Source: CAD feature listing. Evaluate the final solid. Frame: model axes, mm. A direction names the side the tool comes from. Round coordinates to 2 decimals unless told otherwise and drop trailing zeros. Loops run counter-clockwise (first coordinate to the right, second up) from the corner with the lowest first, then second, coordinate; pieces in that order, holes last. Notation, with made-up numbers: (49.5, 84) -> (57.5, 84) arc R23 cw to (57.5, 103) -> close; hole circle Ø10 at (10, 83.25). An arc over 180 degrees is marked (long way). Write item = value, one per line.
Autodesk Inventor part; units mm, degrees
ref_plane "YZ Plane" through (0, 0, 0) normal (1, 0, 0) x (0, 1, 0)
ref_plane "XZ Plane" through (0, 0, 0) normal (0, 1, 0) x (-1, 0, 0)
ref_plane "XY Plane" through (0, 0, 0) normal (0, 0, 1) x (1, 0, 0)
sketch "Sketch1" plane through (0, 0, 0) normal (0, 0, 1) x (1, 0, 0)
  line L0 (-121.92, 53.34) -> (121.92, 53.34)
  line L1 (121.92, 53.34) -> (121.92, -53.34)
  line L2 (121.92, -53.34) -> (-121.92, -53.34)
  line L3 (-121.92, -53.34) -> (-121.92, 53.34)
  line L4 (-121.92, 53.34) -> (121.92, -53.34) construction
  line L5 (121.92, 53.34) -> (-121.92, -53.34) construction
  line L6 (99.0307, 67.3864) -> (98.1801, -71.8373) construction
  line L7 (98.1801, -71.8373) -> (-108.1272, -70.5768) construction
  line L8 (-108.1272, -70.5768) -> (-107.2765, 68.6469) construction
  line L9 (-107.2765, 68.6469) -> (99.0307, 67.3864) construction
  arc A0 (-78.8873, -40.6173) -> (-95.4767, -51.4852) centre (-84.9112, -49.5176) ccw
  arc A1 (-78.8873, -40.6173) -> (-56.3395, -33.0982) centre (-70.4947, -28.2175) ccw
  arc A2 (-36.1227, -22.9374) -> (-56.3395, -33.0982) centre (-42.6558, -35.1316) ccw
  arc A3 (-19.5186, -13.8085) -> (-36.1227, -22.9374) centre (-17.295, -37.5173) ccw
  arc A4 (-68.7224, -13.6289) -> (-40.5344, -17.4333) centre (-51.1537, 10.214) ccw
  arc A5 (-68.7224, -13.6289) -> (-83.4187, -26.4721) centre (-67.6747, -29.6577) ccw
  arc A6 (-92.1839, -37.2444) -> (-83.4187, -26.4721) centre (-103.1345, -19.3818) ccw
  arc A7 (-92.1839, -37.2444) -> (-99.3105, -45.0028) centre (-83.147, -52.6977) ccw
  arc A8 (-99.3105, -45.0028) -> (-95.4767, -51.4852) centre (-95.2121, -46.9539) ccw
  arc A9 (-82.2314, -34.4993) -> (-57.5296, -25.5657) centre (-70.7814, -27.5415) ccw
  arc A10 (-57.5296, -25.5657) -> (-82.2314, -34.4993) centre (-69.6152, -30.7661) ccw
  line L10 (5.4328, -6.7323) -> (-19.5186, -13.8085)
  line L11 (5.4328, -6.7323) -> (85.4483, -20.8459)
  line L12 (85.4483, -20.8459) -> (85.8807, -18.3941)
  line L13 (85.8807, -18.3941) -> (26.167, -0.0762)
  line L14 (26.167, -0.0762) -> (86.2931, 21.1025)
  line L15 (86.2931, 21.1025) -> (85.711, 23.1551)
  arc A11 (85.711, 23.1551) -> (3.7291, 6.4763) centre (298.902, -1234.5808) ccw
  line L16 (-54.4933, 26.4309) -> (-67.6017, 26.4309)
  line L17 (-67.6017, 26.4309) -> (-72.6264, 27.9793)
  line L18 (-72.6264, 27.9793) -> (-69.6152, 32.3411)
  line L19 (-69.6152, 32.3411) -> (-69.6152, 41.676)
  arc A12 (-43.7838, 43.5271) -> (-69.6152, 41.676) centre (-56.4305, 38.848) ccw
  arc A13 (-47.6138, 46.2719) -> (-67.6017, 37.0085) centre (-56.174, 38.5465) ccw
  arc A14 (-67.6017, 37.0085) -> (-47.6138, 46.2719) centre (-56.6407, 39.5536) ccw
  arc A15 (-42.5631, 37.0085) -> (-43.7838, 43.5271) centre (-53.7825, 38.2811) ccw
  arc A16 (-42.5631, 37.0085) -> (-34.9749, 24.888) centre (-24.5395, 39.8568) ccw
  line L20 (-54.4933, 26.4309) -> (-47.0393, 26.4309)
  arc A17 (-36.0743, 21.1026) -> (-47.0393, 26.4309) centre (-51.4449, 3.4184) ccw
  arc A18 (-22.5276, 8.9937) -> (-36.0743, 21.1026) centre (-88.9207, -51.6509) ccw
  arc A19 (-34.9749, 24.888) -> (-17.1938, 11.6747) centre (31.7815, 96.1512) ccw
  line L21 (-22.5276, 8.9937) -> (-16.445, 0)
  line L22 (-16.445, 0) -> (-22.747, -9.6513)
  line L23 (-22.747, -9.6513) -> (-40.5344, -17.4333)
  line L24 (-17.1938, 11.6747) -> (3.7291, 6.4763)
  line L25 (-16.445, 0) -> (3.7291, 6.4763)
  line L26 (5.4328, -6.7323) -> (26.167, -0.0762)
  line L27 (2.2389, 4.8137) -> (6.6839, 4.8137)
  line L28 (6.6839, 4.8137) -> (6.6839, -5.3463)
  line L29 (6.6839, -5.3463) -> (2.2389, -5.3463)
  line L30 (2.2389, -5.3463) -> (2.2389, 4.8137)
  line L31 (2.2389, 4.8137) -> (6.6839, -5.3463) construction
  line L32 (6.6839, 4.8137) -> (2.2389, -5.3463) construction
  point P0 (0, 0)
  point P1 (4.4614, -0.2663)
  dimension "d0" = 243.84
  dimension "d1" = 106.68
  dimension "d23" = 4.445
  dimension "d24" = 10.16
extrude "Extrusion2" add sketch "Sketch1" along normal blind 2.54 contours A0 A8 A7 A6 A5 A4 L23 L22 L25 A11 L15 L14 L26 L10 A3 A2 A1 | L26 L13 L12 L11 | L21 A18 A17 L20 L16 L17 L18 L19 A12 A15 A16 A19 L24 L25
properties part number "RTS Scissors"
1. Section query B-B (z = 1.5). Give the number of separate pieces and of enclosed holes in the cut face, then the cut area to 3 significant figures.
Evaluation:
separate_pieces = 1
enclosed_holes = 3
area = 2,470 mm²
2. Section query A-A (x = -53). Return the cut outline in (y, z) (3 decimals).
Evaluation:
outline = (-25.946, 0) -> (-19.345, 0) -> (-19.345, 2.54) -> (-25.946, 2.54) -> close; (26.431, 0) -> (28.906, 0) -> (28.906, 2.54) -> (26.431, 2.54) -> close; (49.632, 0) -> (51.889, 0) -> (51.889, 2.54) -> (49.632, 2.54) -> close
3. Mould query, pull axis X, two halves, no side actions, for faces 4 (the face through (-74.35, -18.49, 1.25)), 5 (the face through (56.442, -9.363, 1.252)), 6 (the face through (-99.1, -49.3, 1.3)). Classes: released by +X, released by -X, zero draft, split by the parting line, or undercut.
Evaluation:
face_4 = undercut
face_5 = released by +X
face_6 = released by -X
4. Set-up query: faces 1 (the face through (-29.089, 15.476, 1.252)), 2 (the face through (-54.909, -19.164, 1.252)), 3 (the face through (44.88, -13.69, 1.25)). Return all of +Z, -Z, +X, -X, +Y, -Y with unobstructed straight access to the full face (end or side cutting, diameter ignored); none if empty.
Evaluation:
face_1 = +Z, -Z, -X
face_2 = +Z, -Z
face_3 = +Z, -Z, -Y
5. Line query: probe 1 along Y at (x, z) = (43, 0.5); probe 2 along Y at (x, z) = (-26.5, 2) (3 decimals); probe 3 along Y at (x, z) = (-70, 1.1). Output: solid intervals per line, ascending. Write a range as from..to.
Evaluation:
probe_1 = -13.36..-5.24, 5.85..15.16
probe_2 = -15.556..-11.293, 13.075..17.805
probe_3 = -43.18..-40.92, -17.61..-13.76, 27.17..31.78
6. Contact query for flat-ended pins moving along their axis: pin 1 Ø1.3 at (y, z) = (-0.5, 1) entering from -X; pin 2 Ø1.3 at (x, z) = (5, 1.5) entering from -Y; pin 3 Ø0.8 at (x, z) = (4, 1.5) entering from +Y. Output: stop coordinate, or through.
Evaluation:
pin_1 = -17.2
pin_2 = -7.04
pin_3 = 6.64
7. Section query C-C (x = -4). Return the cut outline in (y, z), then the cut area to 3 significant figures.
Evaluation:
outline = (-9.41, 0) -> (8.4, 0) -> (8.4, 2.54) -> (-9.41, 2.54) -> close
area = 45.2 mm²
